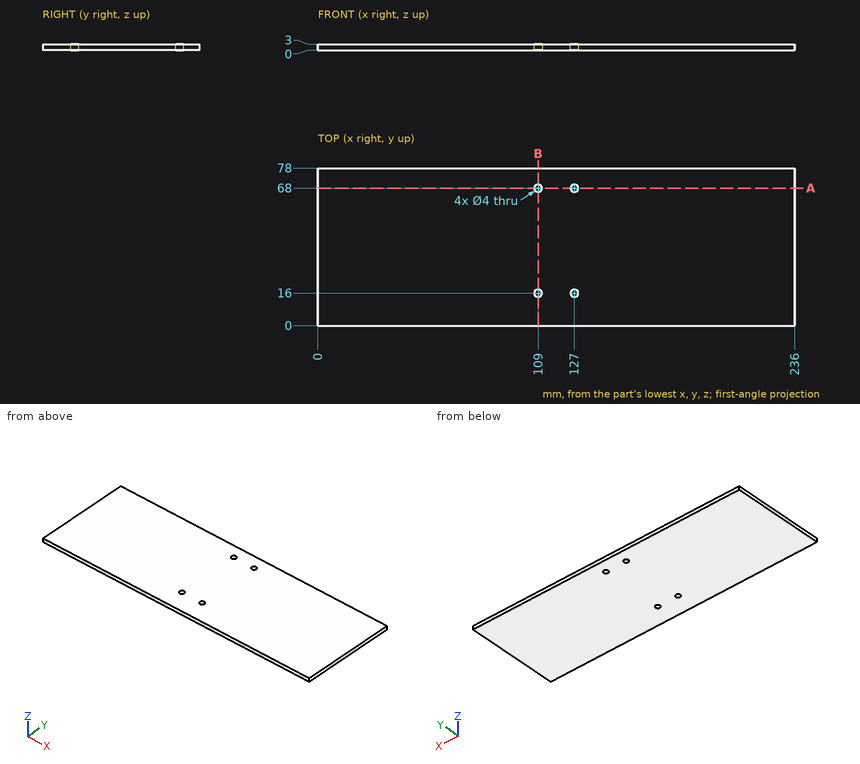
Print and shaded views of the part. All mm, measured from the part's lowest x, y and z. Give positions to 0.01 mm unless a question says otherwise; leave off trailing zeros. Loops run counter-clockwise (first coordinate to the right, second up) from the corner with the lowest first, then second, coordinate; pieces in that order, holes last.
1) Saw through at B-B (x = 109). Write the cut outline in (y, z), plus the area to 3 significant figures.
2) Flat gauge pins, fed straight in: pin 1 Ø4.5 at (x, y) = (109, 16) entering from -Z; pin 2 Ø3 at (x, y) = (109, 68) entering from +Z. Where does each tip first touch, or does it go through?
3) Saw through at A-A (y = 68). Write the cut outline in (x, z), plus the area to 3 significant figures.
4) Wall check: line 1 (Y direction, x = 109, z = 0.95); line 2 (X direction, y = 68, z = 2.05); line 3 (X direction, y = 14.5, z = 0.8). Give the ranges that are in metal, low to high.
Answer block:
1. outline: (0, 0) - (14, 0) - (14, 3) - (0, 3) - close; (18, 0) - (66, 0) - (66, 3) - (18, 3) - close; (70, 0) - (78, 0) - (78, 3) - (70, 3) - close
1. area: 210 mm2
2. pin 1: stops at z = 0
2. pin 2: passes through
3. outline: (0, 0) - (107, 0) - (107, 3) - (0, 3) - close; (111, 0) - (125, 0) - (125, 3) - (111, 3) - close; (129, 0) - (236, 0) - (236, 3) - (129, 3) - close
3. area: 684 mm2
4. line 1: y = 0 to 14, 18 to 66, 70 to 78
4. line 2: x = 0 to 107, 111 to 125, 129 to 236
4. line 3: x = 0 to 107.68, 110.32 to 125.68, 128.32 to 236
